from build123d import *

# Parameters (mm, degrees)
CHANFREIN1_SIZE = 0.5
CHANFREIN2_SIZE = 0.5
CHANFREIN3_SIZE = 0.5


with BuildPart() as part:
    # Esquisse1 → Révolution1 (revolve)
    with BuildSketch(Plane.XY, mode=Mode.PRIVATE) as r_volution1_sk:
        Polygon((0, 0), (0, 9), (-4, 9), (-4, 6), (-16, 6), (-16, 4), (-25, 4), (-25, 3), (-25, 2.5), (-27, 2.5), (-27, 3), (-37, 3), (-37, 0), align=None)
    revolve(r_volution1_sk.sketch.rotate(Axis((-37, 0, 0), (1, 0, 0)), 90), axis=Axis((-37, 0, 0), (1, 0, 0)))  # turned: the seam where the file's is

    # Chanfrein1
    chanfrein1_edges = [part.edges().sort_by_distance(p)[0] for p in [
        (-37, 0, -3),
    ]]
    chamfer(chanfrein1_edges, length=CHANFREIN1_SIZE)

    # Chanfrein2
    chanfrein2_edges = [part.edges().sort_by_distance(p)[0] for p in [
        (-16, 0, -6),
    ]]
    chamfer(chanfrein2_edges, length=CHANFREIN2_SIZE)

    # Chanfrein3
    chanfrein3_edges = [part.edges().sort_by_distance(p)[0] for p in [
        (-25, 0, -4),
    ]]
    chamfer(chanfrein3_edges, length=CHANFREIN3_SIZE)


solid = part.part
Input: part model. Units: mm. Frame: model coordinates. A direction names the side the tool comes from. Give positions to 0.01 mm unless a question says otherwise; leave off trailing zeros. Order: outer loops, then holes, each group sorted by start corner. A loop starts at its lowest first (then second) coordinate and runs counter-clockwise, first axis right, second up. Notation, with made-up numbers: M 31.5,72.5 L 75.5,72.5 A28 ccw 75.5,92.5 Z; hole C 74.5,-16.75 d3. An arc over 180 degrees is marked long. Answer as a JSON object with one key per item and string values.
1. Cut plane D-D, the plane y = 7.5. Output: boundary loops of the cut face in (x, z).
Result sheet:
{"outline": "M -4,-4.97 L 0,-4.97 L 0,4.97 L -4,4.97 Z"}
2. Cut plane A-A, the plane y = 0. Output: boundary loops of the cut face in (x, z).
Result sheet:
{"outline": "M -37,-2.5 L -36.5,-3 L -27,-3 L -27,-2.5 L -25,-2.5 L -25,-3.5 L -24.5,-4 L -16,-4 L -16,-5.5 L -15.5,-6 L -4,-6 L -4,-9 L 0,-9 L 0,9 L -4,9 L -4,6 L -15.5,6 L -16,5.5 L -16,4 L -24.5,4 L -25,3.5 L -25,2.5 L -27,2.5 L -27,3 L -36.5,3 L -37,2.5 Z"}
3. Reachability of faces 5 (the cylindrical face through (-26, -0.1, -2.5)), 6 (the cylindrical face through (-20.31, 3.905, -0.867)), 7 (the flat face through (-37, 0, 0)) from +Z, -Z, +X, -X, +Y, -Y: full face, straight path, thin tool, end or side. Return the list, or none.
Result sheet:
{"face 5": "none", "face 6": "-X", "face 7": "+Z, -Z, -X, +Y, -Y"}
4. Pull-direction query (X, two-part tool) for faces 1 (the cylindrical face through (-2.028, -6.083, -6.633)), 2 (the flat face through (-25, 2, 2)), 3 (the flat face through (-27, -2, 2)), 4 (the flat face through (0, 0, 0)); classes: +X half, -X half, draft (parallel to the pull), parting line (faces both ways), or undercut.
Result sheet:
{"face 1": "draft", "face 2": "undercut", "face 3": "undercut", "face 4": "+X half"}
5. Cut plane C-C, the plane x = -23.5. Output: boundary loops of the cut face in (y, z), and give its area (3 significant figures).
Result sheet:
{"outline": "C 0,0 d8", "area": "50.3 mm²"}
6. Ray query, line 1 (X direction, y = 2.75, z = -6); line 2 (X direction, y = -3, z = 1.25); line 3 (Z direction, x = -6.5, y = 2.75). Return the intervals inside material, ascending. Write a range as [from, to].
Result sheet:
{"line 1": "[-4, 0]", "line 2": "[-25, 0]", "line 3": "[-5.33, 5.33]"}
7. First-contact query: P1, Ø8, axis at x = -10, y = -1.5, coming from the +Z side; P2, Ø5, axis at y = -1.5, z = 0, coming from the +X side; P3, Ø6, axis at x = -28, y = 5.5, coming from the +Z side; P4, Ø2, axis at x = -18.5, y = 4.5, coming from the -Z side. Flat tips, straight axial feed; report the tip coordinate or a pass-through.
Result sheet:
{"P1": "z = 6", "P2": "x = 0", "P3": "z = 1.66", "P4": "z = -1.94"}
